```python
from build123d import *

# Parameters (mm, degrees)
F0_W         = 390
F0_H         = 135
F1_DEPTH     = 590
F2_W         = 384.5905684095
F2_H         = 585
F3_DEPTH     = 132.5
F5_DEPTH     = 590
F7_DEPTH     = 133
F8_T1_DEPTH  = 352.5
F8_T3_DEPTH  = 353.8893095672
F8_T5_DEPTH  = 353.8893095672
F8_T7_DEPTH  = 352.5
F10_DEPTH    = 133
F11_T1_DEPTH = 352.5
F11_T3_DEPTH = 353.8893095672
F11_T5_DEPTH = 353.8893095672
F11_T7_DEPTH = 352.5


# Not quite as in the source:
# - a fillet or chamfer that OpenCascade refuses, or shapes differently, is made with other operations: its cross-section is extruded or revolved along the edge and cut away or added


with BuildPart() as f1:
    # F0 (on Front) → F1 (new body)
    with BuildSketch(Plane.XZ):
        Rectangle(F0_W, F0_H)
    extrude(amount=-F1_DEPTH)

    # F2 (on face) → F3 (cut)
    with BuildSketch(Plane.XY.offset(67.5)):
        with Locations((0, 295)):
            Rectangle(F2_W, F2_H)
    extrude(amount=-F3_DEPTH, mode=Mode.SUBTRACT)

    # F4 (on face) → F5 (join)
    with BuildSketch(Plane.XZ):
        Polygon((-195, 67.5), (-191.1106904328, 67.5), (-342.771697384, 194.7586949967), (-344.3786664082, 192.8435838889), align=None)
        Polygon((191.1106904328, 67.5), (195, 67.5), (344.3786664082, 192.8435838889), (342.771697384, 194.7586949967), align=None)
    extrude(amount=-F5_DEPTH)

    # F6 (on face) → F7 (join)
    with BuildSketch(Plane(origin=(0, 590, 0), x_dir=(-1, 0, 0), z_dir=(0, 1, 0))):
        Polygon((195, 67.5), (344.3786664082, 192.8435838889), (342.771697384, 194.7586949967), (191.1106904328, 67.5), align=None)
        Polygon((-344.3786664082, 192.8435838889), (-195, 67.5), (-191.1106904328, 67.5), (-342.771697384, 194.7586949967), align=None)
    extrude(amount=F7_DEPTH)

    # F8: fillet of radius 70 on 4 edges, made by hand

    # F8_s2 → F8_t1 (cut)
    with BuildSketch(Plane(origin=(-66.762759706, 0, 79.5647587312), x_dir=(0, 1, 0), z_dir=(0.6427876097, 0, -0.7660444431))):
        with BuildLine():
            ThreePointArc((723, 317.766830062), (702.4974746831, 367.2643047451), (653, 387.766830062))
            Line((653, 387.766830062), (723, 387.766830062))
            Line((723, 387.766830062), (723, 317.766830062))
        make_face()
    extrude(amount=F8_T1_DEPTH, mode=Mode.SUBTRACT)

    # F8_s4 → F8_t3 (cut)
    with BuildSketch(Plane.YZ.offset(16.1106904328)):
        with BuildLine():
            ThreePointArc((653, 67.5), (702.4974746831, 88.0025253169), (723, 137.5))
            Line((723, 137.5), (723, 67.5))
            Line((723, 67.5), (653, 67.5))
        make_face()
    extrude(amount=F8_T3_DEPTH, mode=Mode.SUBTRACT)

    # F8_s6 → F8_t5 (cut)
    with BuildSketch(Plane.YZ.offset(-370)):
        with BuildLine():
            ThreePointArc((723, 137.5), (702.4974746831, 88.0025253169), (653, 67.5))
            Line((653, 67.5), (723, 67.5))
            Line((723, 67.5), (723, 137.5))
        make_face()
    extrude(amount=F8_T5_DEPTH, mode=Mode.SUBTRACT)

    # F8_s8 → F8_t7 (cut)
    with BuildSketch(Plane(origin=(-159.8198727085, 0, -190.4659074683), x_dir=(0, 1, 0), z_dir=(0.6427876097, 0, 0.7660444431))):
        with BuildLine():
            ThreePointArc((653, 387.766830062), (702.4974746831, 367.2643047451), (723, 317.766830062))
            Line((723, 317.766830062), (723, 387.766830062))
            Line((723, 387.766830062), (653, 387.766830062))
        make_face()
    extrude(amount=F8_T7_DEPTH, mode=Mode.SUBTRACT)

    # F9 (on face) → F10 (join)
    with BuildSketch(Plane.XZ):
        Polygon((342.771697384, 194.7586949967), (191.1106904328, 67.5), (195, 67.5), (344.3786664082, 192.8435838889), align=None)
        Polygon((-195, 67.5), (-191.1106904328, 67.5), (-342.771697384, 194.7586949967), (-344.3786664082, 192.8435838889), align=None)
    extrude(amount=F10_DEPTH)

    # F11: fillet of radius 70 on 4 edges, made by hand

    # F11_s2 → F11_t1 (cut)
    with BuildSketch(Plane(origin=(66.762759706, 0, 79.5647587312), x_dir=(0, 1, 0), z_dir=(-0.6427876097, 0, -0.7660444431))):
        with BuildLine():
            ThreePointArc((-63, -387.766830062), (-112.4974746831, -367.2643047451), (-133, -317.766830062))
            Line((-133, -317.766830062), (-133, -387.766830062))
            Line((-133, -387.766830062), (-63, -387.766830062))
        make_face()
    extrude(amount=F11_T1_DEPTH, mode=Mode.SUBTRACT)

    # F11_s4 → F11_t3 (cut)
    with BuildSketch(Plane.YZ.offset(-370)):
        with BuildLine():
            ThreePointArc((-133, 137.5), (-112.4974746831, 88.0025253169), (-63, 67.5))
            Line((-63, 67.5), (-133, 67.5))
            Line((-133, 67.5), (-133, 137.5))
        make_face()
    extrude(amount=F11_T3_DEPTH, mode=Mode.SUBTRACT)

    # F11_s6 → F11_t5 (cut)
    with BuildSketch(Plane.YZ.offset(16.1106904328)):
        with BuildLine():
            ThreePointArc((-63, 67.5), (-112.4974746831, 88.0025253169), (-133, 137.5))
            Line((-133, 137.5), (-133, 67.5))
            Line((-133, 67.5), (-63, 67.5))
        make_face()
    extrude(amount=F11_T5_DEPTH, mode=Mode.SUBTRACT)

    # F11_s8 → F11_t7 (cut)
    with BuildSketch(Plane(origin=(159.8198727085, 0, -190.4659074683), x_dir=(0, 1, 0), z_dir=(-0.6427876097, 0, 0.7660444431))):
        with BuildLine():
            ThreePointArc((-133, -317.766830062), (-112.4974746831, -367.2643047451), (-63, -387.766830062))
            Line((-63, -387.766830062), (-133, -387.766830062))
            Line((-133, -387.766830062), (-133, -317.766830062))
        make_face()
    extrude(amount=F11_T7_DEPTH, mode=Mode.SUBTRACT)


solid = f1.part
```
The model under review builds one solid part; all positions refer to its coordinate system, in mm. A direction names the side the tool comes from. Give positions to 0.01 mm unless a question says otherwise; leave off trailing zeros. Write each loop counter-clockwise with the first axis right and the second up, starting at its lowest first coordinate (ties: lowest second). Pieces come first, ordered by that corner, then holes. Notation, with made-up numbers: M -26.5,-39.5 L 23.5,-39.5 A7 cw 23.5,-29.5 Z; hole C 3,-29 d5. An arc over 180 degrees is marked long. Answer in a Markdown table with one row per item.
Item 1: For line 1 along Y through (x, z) = (174, 55); line 2 along X through (y, z) = (380, -39.5); line 3 along Z through (x, y) = (-117.5, 243.5), list the stretches that pass through material, from the lowest coordinate up.
Check sheet entries:
| item | result |
|---|---|
| line 1 | 0 to 2.5, 587.5 to 590 |
| line 2 | -195 to -192.3, 192.3 to 195 |
| line 3 | -67.5 to -65 |
Item 2: Add section C-C on z = -50. Give the boundary of the cut face in (x, y).
Check sheet entries:
| item | result |
|---|---|
| outline | M -195,0 L 195,0 L 195,590 L -195,590 Z; hole M -192.3,2.5 L 192.3,2.5 L 192.3,587.5 L -192.3,587.5 Z |
Item 3: Add section A-A on y = 642. Give the boundary of the cut face in (x, z), plus the area to 3 significant figures.
Check sheet entries:
| item | result |
|---|---|
| outline | M -344.38,192.84 L -195,67.5 L -191.11,67.5 L -342.77,194.76 Z; M 191.11,67.5 L 195,67.5 L 344.38,192.84 L 342.77,194.76 Z |
| area | 982 mm2 |
Item 4: Tool access review of faces 1 (the face through (268, 300.99, 132.02)), 2 (the face through (-218.802, -112.679, 88.184)), 3 (the face through (192.295, 291, 2)): name each direction out of +Z, -Z, +X, -X, +Y, -Y from which nothing blocks a thin tool from reaching the whole face with its end or side.
Check sheet entries:
| item | result |
|---|---|
| face 1 | +Z, +Y, -Y |
| face 2 | -Z, +X, -X, -Y |
| face 3 | none |
Item 5: For P1, Ø8, axis at y = 165, z = 87.5, coming from the -X side; P2, Ø1.2, axis at x = -192.5, y = 623.5, coming from the -Z side; P3, Ø2, axis at x = -9, y = 589, coming from the +Z side, all flat-tipped, find the tip position at first contact; note any pin that passes through.
Check sheet entries:
| item | result |
|---|---|
| P1 | x = -223.6 |
| P2 | z = 67.5 |
| P3 | z = 67.5 |
Item 6: Add section D-D on x = 150. Give the boundary of the cut face in (y, z).
Check sheet entries:
| item | result |
|---|---|
| outline | M 0,-67.5 L 590,-67.5 L 590,67.5 L 587.5,67.5 L 587.5,-65 L 2.5,-65 L 2.5,67.5 L 0,67.5 Z |
Item 7: Add section B-B on z = 109.5. Give the boundary of the cut face in (x, y), plus the area to 3 significant figures.
Check sheet entries:
| item | result |
|---|---|
| outline | M -245.05,-127.16 L -241.16,-127.16 L -241.16,717.16 L -245.05,717.16 Z; M 241.16,-127.16 L 245.05,-127.16 L 245.05,717.16 L 241.16,717.16 Z |
| area | 6,570 mm2 |
Item 8: Draft analysis for pull direction X (two halves, no side actions). For faces 4 (the face through (-3, 590, 1)), 5 (the face through (-192.295, 291, 2)), 6 (the face through (-195, 291, -1)), 7 (the face through (327.44, 703.04, 180.28)), state which applies: +X half, -X half, draft (parallel to the pull), parting line (faces both ways), or undercut.
Check sheet entries:
| item | result |
|---|---|
| face 4 | draft |
| face 5 | undercut |
| face 6 | -X half |
| face 7 | +X half |
